```python
from build123d import *

# Parameters (mm, degrees)
SKETCH_1_R                           = 8.5
EXTRUDE_537_DEPTH                    = 28
SKETCH_2_R                           = 10
EXTRUDE_624_DEPTH                    = 3
EXTRUDE_747_DEPTH                    = 5
SKETCH_4_R                           = 3.15
CUT_EXTRUDE_845_DEPTH                = 12
SKETCH_5_W                           = 2.3
SKETCH_5_H                           = 7.5
CUT_EXTRUDE_1044_DEPTH               = 10
SKETCH_6_R                           = 2.2
CUT_EXTRUDE_1_DEPTH                  = 40.676472878
CUT_EXTRUDE_1_DIRECTION_2_REACH      = 41.676
CUT_EXTRUDE_1_DIRECTION_2_END_RADIUS = 3.15
SKETCH_7_R                           = 2.2
CUT_EXTRUDE_2_DEPTH                  = 40.984324454
CUT_EXTRUDE_2_DIRECTION_2_REACH      = 41.984
CUT_EXTRUDE_2_DIRECTION_2_END_RADIUS = 3.15
SKETCH_10_R                          = 1.75
CUT_EXTRUDE_1470_DEPTH               = 39.678159305


with BuildPart() as part:
    # Эскиз1 → Extrude 537 (new body)
    with BuildSketch(Plane(origin=(0, 0, 0), x_dir=(1, 0, 0), z_dir=(0, 1, 0))):
        with Locations(Location((0, 0, 0), (0, 0, 270))):
            Circle(SKETCH_1_R)
    extrude(amount=EXTRUDE_537_DEPTH)

    # Эскиз2 → Extrude 624 (add)
    with BuildSketch(Plane(origin=(0, 28, 0), x_dir=(1, 0, 0), z_dir=(0, 1, 0))):
        with Locations(Location((0, 0, 0), (0, 0, 270))):
            Circle(SKETCH_2_R)
    extrude(amount=EXTRUDE_624_DEPTH)

    # Эскиз3 → Extrude 747 (add)
    with BuildSketch(Plane(origin=(0, 31, 0), x_dir=(1, 0, 0), z_dir=(0, 1, 0))):
        Polygon((9.988159657, 0), (4.994079828, 8.65), (-4.994079828, 8.65), (-9.988159657, 0), (-4.994079828, -8.65), (4.994079828, -8.65), align=None)
    extrude(amount=EXTRUDE_747_DEPTH)

    # Эскиз4 → Cut-Extrude 845 (cut)
    with BuildSketch(Plane.XZ):
        with Locations(Location((0, 0, 0), (0, 0, 270))):
            Circle(SKETCH_4_R)
    extrude(amount=-CUT_EXTRUDE_845_DEPTH, mode=Mode.SUBTRACT)

    # Эскиз5 → Cut-Extrude 1044 (cut)
    with BuildSketch(Plane.XZ):
        with Locations((4.5, 0)):
            Rectangle(SKETCH_5_W, SKETCH_5_H)
        Polygon((-4.922595264, -1.026185103), (1.572595264, -4.776185103), (0.422595264, -6.768043531), (-6.072595264, -3.018043531), align=None)
    extrude(amount=-CUT_EXTRUDE_1044_DEPTH, mode=Mode.SUBTRACT)

    # Эскиз6 → отверстие чтоб прикрутить 1 (cut)
    with BuildSketch(Plane(origin=(3.35, 0, 0), x_dir=(0, 0, -1), z_dir=(1, 0, 0))):
        with Locations(Location((0, 4.5, 0), (0, 0, 180))):
            Circle(SKETCH_6_R)
    extrude(amount=CUT_EXTRUDE_1_DEPTH, mode=Mode.SUBTRACT)

    # отверстие чтоб прикрутить 1 direction 2: up to this cylinder (the profile starts outside it)
    cut_extrude_1_direction_2_end = Plane(origin=(0, 4.5, 0), z_dir=(0, -1, 0)) * Cylinder(CUT_EXTRUDE_1_DIRECTION_2_END_RADIUS, 90.652, mode=Mode.PRIVATE)
    # Эскиз6 → отверстие чтоб прикрутить 1 direction 2 (cut, up to the surface)
    with BuildSketch(Plane(origin=(3.35, 0, 0), x_dir=(0, 0, -1), z_dir=(1, 0, 0)), mode=Mode.PRIVATE) as cut_extrude_1_direction_2_sk1:
        with Locations(Location((0, 4.5, 0), (0, 0, 180))):
            Circle(SKETCH_6_R)
    cut_extrude_1_direction_2_tool1 = extrude(cut_extrude_1_direction_2_sk1.sketch, amount=-CUT_EXTRUDE_1_DIRECTION_2_REACH, mode=Mode.PRIVATE) - cut_extrude_1_direction_2_end
    add(cut_extrude_1_direction_2_tool1.solids().sort_by_distance((3.35, 4.5, 0))[0], mode=Mode.SUBTRACT)

    # Эскиз7 → отверстие чтоб прикрутить 2 (cut)
    with BuildSketch(Plane(origin=(-1.675, 0, -2.901185103), x_dir=(-0.8660254037844362, 0, 0.5000000000000042), z_dir=(-0.5000000000000043, 0, -0.8660254037844363))):
        with Locations(Location((0, 4.5, 0), (0, 0, 180))):
            Circle(SKETCH_7_R)
    extrude(amount=CUT_EXTRUDE_2_DEPTH, mode=Mode.SUBTRACT)

    # отверстие чтоб прикрутить 2 direction 2: up to this cylinder (the profile starts outside it)
    cut_extrude_2_direction_2_end = Plane(origin=(0, 4.5, 0), z_dir=(0, -1, 0)) * Cylinder(CUT_EXTRUDE_2_DIRECTION_2_END_RADIUS, 91.268, mode=Mode.PRIVATE)
    # Эскиз7 → отверстие чтоб прикрутить 2 direction 2 (cut, up to the surface)
    with BuildSketch(Plane(origin=(-1.675, 0, -2.901185103), x_dir=(-0.8660254037844362, 0, 0.5000000000000042), z_dir=(-0.5000000000000043, 0, -0.8660254037844363)), mode=Mode.PRIVATE) as cut_extrude_2_direction_2_sk1:
        with Locations(Location((0, 4.5, 0), (0, 0, 180))):
            Circle(SKETCH_7_R)
    cut_extrude_2_direction_2_tool1 = extrude(cut_extrude_2_direction_2_sk1.sketch, amount=-CUT_EXTRUDE_2_DIRECTION_2_REACH, mode=Mode.PRIVATE) - cut_extrude_2_direction_2_end
    add(cut_extrude_2_direction_2_tool1.solids().sort_by_distance((-1.675, 4.5, -2.901185))[0], mode=Mode.SUBTRACT)

    # Эскиз10 → Cut-Extrude 1470 (cut, through all)
    with BuildSketch(Plane(origin=(0, 36, 0), x_dir=(1, 0, 0), z_dir=(0, 1, 0))):
        with Locations(Location((0, 0, 0), (0, 0, 270))):
            Circle(SKETCH_10_R)
    extrude(amount=-CUT_EXTRUDE_1470_DEPTH, mode=Mode.SUBTRACT)


solid = part.part
```
Geometry: final body of the model. Coordinates: model frame, mm. A direction names the side the tool comes from. Round coordinates to 2 decimals unless told otherwise and drop trailing zeros. Write each loop counter-clockwise with the first axis right and the second up, starting at its lowest first coordinate (ties: lowest second). Pieces come first, ordered by that corner, then holes.
Item 1: Section query D-D (y = 30). Return loops of the section in (x, z), plus the area to 3 significant figures.
Item 2: Pin query (flat end, axial travel): P1, Ø10, axis at x = 0, z = 0, coming from the -Y side; P2, Ø1.5, axis at y = 29, z = -6.5, coming from the +X side; P3, Ø1.7, axis at x = -2.5, z = -4, coming from the -Y side; P4, Ø4, axis at x = -2.5, y = 34.5, coming from the -Z side. Return the tip coordinate at first contact, or that it passes through.
Item 3: Section query C-C (y = 4.5). Return loops of the section in (x, z).
Item 4: Section query A-A (y = 15). Return loops of the section in (x, z), plus the area to 3 significant figures.
Item 5: Material intervals for L1, parallel to Y at x = 6.5, z = 0; L2, parallel to X at y = 6, z = 2; L3, parallel to Y at x = 5, z = 1, sorted ascending.
Item 6: Set-up query: faces 5 (the face through (4, 5, 3.75)), 6 (the face through (7.06, 2.32, -0.29)), 7 (the face through (-7.53, 33.47, 4.26)), 8 (the face through (-7.456, 33.465, -4.386)). Return all of +Z, -Z, +X, -X, +Y, -Y with unobstructed straight access to the full face (end or side cutting, diameter ignored); none if empty.
Item 7: Mould query, pull axis Y, two halves, no side actions, for faces 1 (the face through (-1.4, 12, -1.4)), 2 (the face through (0, 31, 9)), 3 (the face through (2.93, 3.84, 2.1)), 4 (the face through (-2.78, 7.15, -4.92)). Classes: +Y half, -Y half, draft (parallel to the pull), parting line (faces both ways), or undercut.
Item 8: Section query B-B (x = -8). Return loops of the section in (y, z), plus the area to 3 significant figures.
Completed:
1. outline: circle Ø20 at (0, 0); hole circle Ø3.5 at (0, 0)
1. area: 305 mm2
2. P1: stops at y = 0
2. P2: stops at x = 8.18
2. P3: stops at y = 10
2. P4: stops at z = -8.65
3. outline: (-6.07, -3.02) - (-4.92, -1.03) - (-3.58, -1.8) - (-3.03, -0.85) arc R3.15 cw to (2.25, 2.2) - (3.35, 2.2) - (3.35, 3.75) - (5.65, 3.75) - (5.65, 2.2) - (8.21, 2.2) arc R8.5 ccw (long way) to (-6.01, -6.01) - (-4.73, -3.79) - close; (-2.2, -8.21) arc R8.5 ccw to (8.21, -2.2) - (5.65, -2.2) - (5.65, -3.75) - (3.35, -3.75) - (3.35, -2.2) - (2.25, -2.2) arc R3.15 cw to (0.78, -3.05) - (0.23, -4) - (1.57, -4.78) - (0.42, -6.77) - (-0.92, -5.99) - close
4. outline: circle Ø17 at (0, 0); hole circle Ø3.5 at (0, 0)
4. area: 217 mm2
5. L1: y = 0 to 2.3, 6.7 to 36
5. L2: x = -8.26 to -2.43, 2.43 to 3.35, 5.65 to 8.26
5. L3: y = 10 to 36
6. face 5: -Y
6. face 6: +X
6. face 7: +Z, -X, +Y
6. face 8: -Z, -X, +Y
7. face 1: -Y half
7. face 2: +Y half
7. face 3: undercut
7. face 4: draft
8. outline: (0, -2.87) - (28, -2.87) - (28, -6) - (31, -6) - (31, -3.44) - (36, -3.44) - (36, 3.44) - (31, 3.44) - (31, 6) - (28, 6) - (28, 2.87) - (0, 2.87) - close
8. area: 231 mm2
